Build history of the part. All positions in model axes, mm. Face numbers are marked on the shaded views. A direction names the side the tool comes from. Give positions to 0.01 mm unless a question says otherwise; leave off trailing zeros. Loops run counter-clockwise (first coordinate to the right, second up) from the corner with the lowest first, then second, coordinate; pieces in that order, holes last. Notation, with made-up numbers: (-27, 7.25) - (17, 7.25) arc R17 cw to (17, 33.25) - close; hole circle Ø8 at (13, 15.25). An arc over 180 degrees is marked (long way). Return JSON: item names as keys, results as strings. Group by question number.
1) Drop flat-ended pins along their axis: pin 1 (5 mm diameter, centred on y = -16, z = 53.5, fed in from -X); pin 2 (5 mm diameter, centred on y = -14, z = 15.5, fed in from -X); pin 3 (21 mm diameter, centred on x = 10.5, y = -4.5, fed in from +Z); pin 4 (18 mm diameter, centred on x = 90, y = 0, fed in from +Z). Give the stop position or say it passes through.
2) 3-axis set-ups, long thin cutter, end or side, ignore diameter. For the marked faces 4, 5, 6 and 7: which of +Z, -Z, +X, -X, +Y, -Y reach the whole face in a straight line?
3) Slice it at A-A (y = 0). List the corners of the cut face in (x, z).
4) Slice it at B-B (z = 56.5). List the corners of the cut face in (x, y), and give its area (3 significant figures).
5) Slice it at C-C (y = 17). List the corners of the cut face in (x, z).
6) Mould opens along Y. For the marked faces 1, 2 and 3 say: released by +Y, released by -Y, zero draft, split by the parting line, or undercut.
7) Slice it at D-D (z = 23.5). List the corners of the cut face in (x, y).
8) Drill centre lines: probe 1 along Y at (x, z) = (90, 31); probe 2 along X at (y, z) = (0, 52.5); probe 3 along Z at (x, y) = (107, 8.5). Where is each one in solid material? Low to high. Write a range as from..to.
```python
from build123d import *

# Parameters (mm, degrees)
BOSS_EXTRUDE1_DEPTH = 70
BOSS_EXTRUDE2_DEPTH = 10
SKETCH3_R           = 30
CUT_EXTRUDE1_DEPTH  = 30
SKETCH4_R           = 10
CUT_EXTRUDE2_DEPTH  = 71
CUT_EXTRUDE6_DEPTH  = 50
SKETCH9_R           = 20
CUT_EXTRUDE7_DEPTH  = 50
CUT_EXTRUDE8_DEPTH  = 20


with BuildPart() as part:
    # Sketch1 → Boss-Extrude1 (new body)
    with BuildSketch(Plane.XY):
        with BuildLine():
            Line((0, 50), (90, 50))
            ThreePointArc((90, 50), (140, 0), (90, -50))
            Line((90, -50), (0, -50))
            ThreePointArc((0, -50), (-50, 0), (0, 50))
        make_face()
    extrude(amount=BOSS_EXTRUDE1_DEPTH)

    # Sketch2 → Boss-Extrude2 (add)
    with BuildSketch(Plane.XY.offset(70)):
        with BuildLine():
            Line((90, 50), (90, 30))
            ThreePointArc((90, 30), (120, 0), (90, -30))
            Line((90, -30), (90, -50))
            ThreePointArc((90, -50), (140, 0), (90, 50))
        make_face()
    extrude(amount=BOSS_EXTRUDE2_DEPTH)

    # Sketch3 → Cut-Extrude1 (cut)
    with BuildSketch(Plane.XY.offset(70)):
        with Locations((90, 0)):
            Circle(SKETCH3_R)
    extrude(amount=-CUT_EXTRUDE1_DEPTH, mode=Mode.SUBTRACT)

    # Sketch4 → Cut-Extrude2 (cut)
    with BuildSketch(Plane.XY.offset(40)):
        with Locations((90, 0)):
            Circle(SKETCH4_R)
    extrude(amount=-CUT_EXTRUDE2_DEPTH, mode=Mode.SUBTRACT)

    # Sketch5 → Cut-Extrude6 (cut)
    with BuildSketch(Plane.XY.offset(70)):
        with BuildLine():
            Line((0, 35), (-35.707142143, 35))
            ThreePointArc((-35.707142143, 35), (-50, 0), (-35.707142143, -35))
            Line((-35.707142143, -35), (0, -35))
            ThreePointArc((0, -35), (35, 0), (0, 35))
        make_face()
    extrude(amount=-CUT_EXTRUDE6_DEPTH, mode=Mode.SUBTRACT)

    # Sketch9 → Cut-Extrude7 (cut)
    with BuildSketch(Plane.XY.offset(20)):
        Circle(SKETCH9_R)
    extrude(amount=-CUT_EXTRUDE7_DEPTH, mode=Mode.SUBTRACT)

    # Sketch10 → Cut-Extrude8 (cut)
    with BuildSketch(Plane.XY.offset(70)):
        with BuildLine():
            ThreePointArc((73.416876048, -25), (60, 0), (73.416876048, 25))
            Line((73.416876048, 25), (24.494897428, 25))
            ThreePointArc((24.494897428, 25), (35, 0), (24.494897428, -25))
            Line((24.494897428, -25), (73.416876048, -25))
        make_face()
    extrude(amount=-CUT_EXTRUDE8_DEPTH, mode=Mode.SUBTRACT)


solid = part.part
```
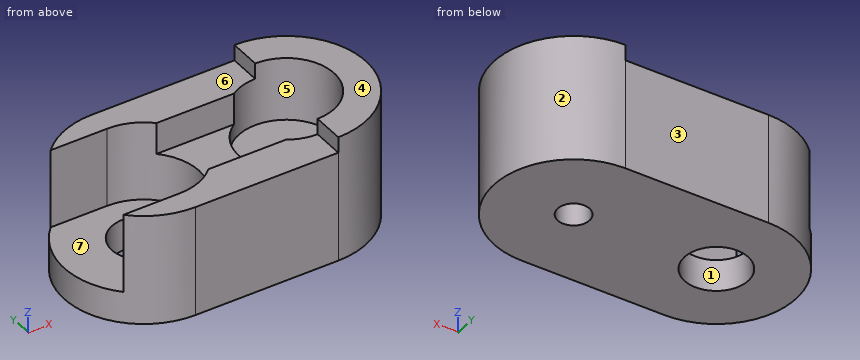
Results:
{
 "1": {"pin 1": "x = 113.62", "pin 2": "x = -48.66", "pin 3": "z = 20", "pin 4": "through"},
 "2": {"face 4": "+Z, +X, -X, +Y, -Y", "face 5": "+Z", "face 6": "+Z, -X, +Y, -Y", "face 7": "+Z, -X"},
 "3": {"outline": "(-50, 0) - (-20, 0) - (-20, 20) - (-50, 20) - close; (20, 0) - (80, 0) - (80, 40) - (60, 40) - (60, 50) - (35, 50) - (35, 20) - (20, 20) - close; (100, 0) - (140, 0) - (140, 80) - (120, 80) - (120, 40) - (100, 40) - close"},
 "4": {"outline": "(-35.71, -35) arc R50 ccw to (0, -50) - (90, -50) arc R50 ccw to (90, 50) - (0, 50) arc R50 ccw to (-35.71, 35) - (0, 35) arc R35 cw to (24.49, 25) - (73.42, 25) arc R30 cw (long way) to (73.42, -25) - (24.49, -25) arc R35 cw to (0, -35) - close", "area": "7,300 mm2"},
 "5": {"outline": "(-47.02, 0) - (-10.54, 0) - (-10.54, 20) - (-47.02, 20) - close; (10.54, 0) - (137.02, 0) - (137.02, 80) - (114.72, 80) - (114.72, 40) - (65.28, 40) - (65.28, 50) - (30.59, 50) - (30.59, 20) - (10.54, 20) - close"},
 "6": {"face 1": "undercut", "face 2": "split by the parting line", "face 3": "released by +Y"},
 "7": {"outline": "(-35.71, -35) arc R50 ccw to (0, -50) - (90, -50) arc R50 ccw to (90, 50) - (0, 50) arc R50 ccw to (-35.71, 35) - (0, 35) arc R35 cw to (0, -35) - close; hole circle Ø20 at (90, 0)"},
 "8": {"probe 1": "-50..-10, 10..50", "probe 2": "120..140", "probe 3": "0..40"}
}
